Verification items for the finished model (mm, model axes). Give positions to 0.01 mm unless a question says otherwise; leave off trailing zeros. Write each loop counter-clockwise with the first axis right and the second up, starting at its lowest first coordinate (ties: lowest second). Pieces come first, ordered by that corner, then holes.
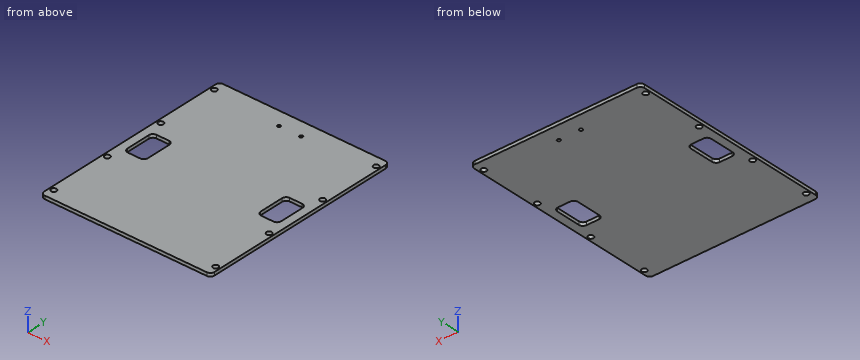
from build123d import *

# Parameters (mm, degrees)
BOARDOUTLINE_DEPTH   = 1.6
SKETCH2_R            = 0.8
COMPONENTHOLES_DEPTH = 2.6
WINDOWS_1SIDE_DEPTH  = 2.6
M2_CLEARANCE_HOLE1_D = 2.6


with BuildPart() as part:
    # Sketch1 → boardOutline (new body)
    with BuildSketch(Plane.XY):
        with BuildLine():
            Line((-39.5, -50), (39.5, -50))
            ThreePointArc((39.5, -50), (40.914213562, -49.414213562), (41.5, -48))
            Line((41.5, -48), (41.5, 48))
            ThreePointArc((41.5, 48), (40.914213562, 49.414213562), (39.5, 50))
            Line((39.5, 50), (-39.5, 50))
            ThreePointArc((-39.5, 50), (-40.914213562, 49.414213562), (-41.5, 48))
            Line((-41.5, 48), (-41.5, -48))
            ThreePointArc((-41.5, -48), (-40.914213562, -49.414213562), (-39.5, -50))
        make_face()
    extrude(amount=BOARDOUTLINE_DEPTH)

    # Sketch2 → componentHoles (cut, through all)
    with BuildSketch(Plane.XY.offset(1.6)):
        with Locations((-5.385, 42.1)):
            Circle(SKETCH2_R)
        with Locations((5.385, 42.1)):
            Circle(SKETCH2_R)
    extrude(amount=-COMPONENTHOLES_DEPTH, mode=Mode.SUBTRACT)

    # Sketch3 → windows_1side (cut, through all)
    with BuildSketch(Plane.XY.offset(1.6)):
        with BuildLine():
            Line((37.5, -6), (37.5, 6))
            ThreePointArc((37.5, 6), (36.914213562, 7.414213562), (35.5, 8))
            Line((35.5, 8), (29.5, 8))
            ThreePointArc((29.5, 8), (28.085786438, 7.414213562), (27.5, 6))
            Line((27.5, 6), (27.5, -6))
            ThreePointArc((27.5, -6), (28.085786438, -7.414213562), (29.5, -8))
            Line((29.5, -8), (35.5, -8))
            ThreePointArc((35.5, -8), (36.914213562, -7.414213562), (37.5, -6))
        make_face()
        with BuildLine():
            Line((-29.5, -8), (-35.5, -8))
            ThreePointArc((-35.5, -8), (-36.914213562, -7.414213562), (-37.5, -6))
            Line((-37.5, -6), (-37.5, 6))
            ThreePointArc((-37.5, 6), (-36.914213562, 7.414213562), (-35.5, 8))
            Line((-35.5, 8), (-29.5, 8))
            ThreePointArc((-29.5, 8), (-28.085786438, 7.414213562), (-27.5, 6))
            Line((-27.5, 6), (-27.5, -6))
            ThreePointArc((-27.5, -6), (-28.085786438, -7.414213562), (-29.5, -8))
        make_face()
    extrude(amount=-WINDOWS_1SIDE_DEPTH, mode=Mode.SUBTRACT)

    # M2 Clearance Hole1 (through all)
    with Locations(Plane(origin=(0, 0, 0), x_dir=(-1, 0, 0), z_dir=(0, 0, -1))):
        with Locations((39.5, 45), (39.5, -15), (39.5, -45), (39.5, 15)):
            m2_clearance_hole1 = Hole(M2_CLEARANCE_HOLE1_D / 2)

    # Mirror1: M2 Clearance Hole1 across plane
    add(m2_clearance_hole1.mirror(Plane(origin=(0, 0, 0), x_dir=(0, 0, 1), z_dir=(1, 0, 0))), mode=Mode.SUBTRACT)


solid = part.part
Item 1: Sectioned sample at C-C on y = 1.5. Record the cut outline in (x, z).
Answer key:
outline: (-41.5, 0) - (-37.5, 0) - (-37.5, 1.6) - (-41.5, 1.6) - close; (-27.5, 0) - (27.5, 0) - (27.5, 1.6) - (-27.5, 1.6) - close; (37.5, 0) - (41.5, 0) - (41.5, 1.6) - (37.5, 1.6) - close
Item 2: Depth check by flat-ended pin: pin 1 (1.6 mm diameter, centred on x = 39.5, y = -45, fed in from +Z). Enter the tip coordinate at first touch or a pass-through.
Answer key:
pin 1: passes through
Item 3: Scan lines: line 1 along X through (y, z) = (42.1, 0.9) (3 decimals); line 2 along X through (y, z) = (-1, 1.55); line 3 along Y through (x, z) = (39.5, 0.35). Record each from-to range of solid material in increasing order.
Answer key:
line 1: x = -41.5 to -6.185, -4.585 to 4.585, 6.185 to 41.5
line 2: x = -41.5 to -37.5, -27.5 to 27.5, 37.5 to 41.5
line 3: y = -50 to -46.3, -43.7 to -16.3, -13.7 to 13.7, 16.3 to 43.7, 46.3 to 50
Item 4: Sectioned sample at B-B on z = 0.85. State how many separate pieces and enclosed holes the cut face has, then the cut area to 3 significant figures.
Answer key:
separate pieces: 1
enclosed holes: 12
area: 7,940 mm2
Item 5: Sectioned sample at A-A on y = 15. Record the cut outline in (x, z), then the cut area to 3 significant figures.
Answer key:
outline: (-41.5, 0) - (-40.8, 0) - (-40.8, 1.6) - (-41.5, 1.6) - close; (-38.2, 0) - (38.2, 0) - (38.2, 1.6) - (-38.2, 1.6) - close; (40.8, 0) - (41.5, 0) - (41.5, 1.6) - (40.8, 1.6) - close
area: 124 mm2
